from build123d import *
from build123d.topology import SkipClean

# Parameters (mm, degrees)
SKETCH1_R                                = 2.5
BOSS_EXTRUDE1_DEPTH                      = 2.5
SKETCH4_W                                = 130
SKETCH4_H                                = 30
BOSS_EXTRUDE2_DEPTH                      = 5
FILLET1_R                                = 10
FILLET2_R                                = 12.5
SKETCH5_R                                = 2.15
CUT_EXTRUDE1_DEPTH                       = 10
BOSS_EXTRUDE3_DEPTH                      = 2.5
LPATTERN1_COUNT                          = 2
LPATTERN1_PITCH                          = 23
MIRROR4_COPY_1_DEPTH                     = 2.5
MIRROR4_AT_THE_SECOND_PLANE_COPY_1_DEPTH = 2.5
MIRROR4_AT_THE_SECOND_PLANE_COPY_2_DEPTH = 2.5
MIRROR4_AT_THE_SECOND_PLANE_COPY_3_DEPTH = 2.5


with BuildPart() as part:
    # Sketch1 → Boss-Extrude1 (new, symmetric)
    with BuildSketch(Plane.XY):
        with BuildLine():
            ThreePointArc((-38.614160498, -3.933326056), (-23.874667518, 3.933250754), (-9.779272654, -5.036449778))
            ThreePointArc((-9.779272654, -5.036449778), (-5.727087063, -9.391510729), (0, -11))
            Line((0, -11), (0, -4))
            ThreePointArc((0, -4), (-4, 0), (0, 4))
            Line((0, 4), (0, 11))
            Line((0, 11), (-52.5, 11))
            Line((-52.5, 11), (-52.5, 0))
            ThreePointArc((-52.5, 0), (-47.044040574, -7.216086067), (-38.614160498, -3.933326056))
        make_face()
        with Locations((-45, 0)):
            Circle(SKETCH1_R, mode=Mode.SUBTRACT)
    boss_extrude1 = extrude(amount=BOSS_EXTRUDE1_DEPTH, both=True)

    # Mirror1: Boss-Extrude1 across plane
    with SkipClean():  # the faces are left unmerged after this step: merging them gives an invalid solid
        add(boss_extrude1.mirror(Plane(origin=(0, 0, -2.5), x_dir=(0, 0, 1), z_dir=(-1, 0, 0))))

    # Sketch4 → Boss-Extrude2 (add)
    with SkipClean():  # the faces are left unmerged after this step: merging them gives an invalid solid
        with BuildSketch(Plane(origin=(0, 11, 0), x_dir=(1, 0, 0), z_dir=(0, 1, 0))):
            Rectangle(SKETCH4_W, SKETCH4_H)
        extrude(amount=BOSS_EXTRUDE2_DEPTH)

    # Fillet1
    fillet1_edges = [part.edges().sort_by_distance(p)[0] for p in [
        (-65, 13.5, -15),
        (-65, 13.5, 15),
        (65, 13.5, 15),
        (65, 13.5, -15),
    ]]
    fillet(fillet1_edges, radius=FILLET1_R)

    # Fillet2
    # the kernel refuses this fillet: 12.5 mm, written as the material it adds along each edge
    with BuildSketch(Plane(origin=(-52.5, 11, -2.5), x_dir=(-1, 0, 0), z_dir=(0, 0, 1))) as fillet2_piece_1:
        with BuildLine():
            CenterArc((12.443670675, 12.5), FILLET2_R, 184.301222305, 85.698777695)
            Line((-0.021123497, 11.5625), (-1.267602914, 11.46875))
            ThreePointArc((-1.267602914, 11.46875), (-1.25, 11), (-1.25, 0))
            Line((-1.25, 0), (0, -1.25))
            Line((0, -1.25), (12.443670675, -1.25))
            Line((12.443670675, -1.25), (12.443670675, 0))
        make_face()
    extrude(amount=5)
    with BuildSketch(Plane(origin=(52.5, 11, -2.5), x_dir=(1, 0, 0), z_dir=(0, 0, 1))) as fillet2_piece_2:
        with BuildLine():
            CenterArc((12.443670675, -12.5), FILLET2_R, 90, 85.698777695)
            Line((-0.021123497, -11.5625), (-1.267602914, -11.46875))
            ThreePointArc((-1.267602914, -11.46875), (-1.25, -11), (-1.25, 0))
            Line((-1.25, 0), (0, 1.25))
            Line((0, 1.25), (12.443670675, 1.25))
            Line((12.443670675, 1.25), (12.443670675, 0))
        make_face()
    extrude(amount=5)

    # Sketch5 → Cut-Extrude1 (cut)
    with BuildSketch(Plane(origin=(0, 16, 0), x_dir=(1, 0, 0), z_dir=(0, 1, 0))):
        with Locations(Location((-57, -8, 0), (0, 0, 180))):
            Circle(SKETCH5_R)
        with Locations(Location((-57, 8, 0), (0, 0, 180))):
            Circle(SKETCH5_R)
        with Locations(Location((-23, -8, 0), (0, 0, 180))):
            Circle(SKETCH5_R)
        with Locations(Location((-23, 8, 0), (0, 0, 180))):
            Circle(SKETCH5_R)
    cut_extrude1 = extrude(amount=-CUT_EXTRUDE1_DEPTH, mode=Mode.SUBTRACT)

    # Mirror2: Cut-Extrude1 across plane
    add(cut_extrude1.mirror(Plane(origin=(0, 0, 0), x_dir=(0, 0, 1), z_dir=(1, 0, 0))), mode=Mode.SUBTRACT)

    # Sketch7 → Boss-Extrude3 (add, symmetric)
    with BuildSketch(Plane(origin=(36.5, 0, 0), x_dir=(0, 0, -1), z_dir=(1, 0, 0))):
        Polygon((5, 11), (2.5, 11), (2.5, 6), (7.5, 11), align=None)
    boss_extrude3 = extrude(amount=BOSS_EXTRUDE3_DEPTH, both=True)

    # LPattern1: Boss-Extrude3 ×2
    with Locations(*[(-i * LPATTERN1_PITCH, 0, 0) for i in range(1, LPATTERN1_COUNT)]):
        add(boss_extrude3)

    # Mirror4: Boss-Extrude3 across plane
    add(boss_extrude3.mirror(Plane.XY))

    # Mirror4 copy 1 sketch → Mirror4 copy 1 (add, symmetric)
    with BuildSketch(Plane(origin=(13.5, 0, 0), x_dir=(0, 0, 1), z_dir=(1, 0, 0))):
        Polygon((5, -11), (2.5, -11), (2.5, -6), (7.5, -11), align=None)
    extrude(amount=MIRROR4_COPY_1_DEPTH, both=True)

    # Mirror4 at the second plane: Boss-Extrude3 across plane
    add(boss_extrude3.mirror(Plane(origin=(0, 0, 0), x_dir=(0, 0, 1), z_dir=(1, 0, 0))))

    # Mirror4 at the second plane copy 1 sketc → Mirror4 at the second plane copy 1 (add, symmetric)
    with BuildSketch(Plane(origin=(-13.5, 0, 0), x_dir=(0, 0, -1), z_dir=(-1, 0, 0))):
        Polygon((5, -11), (2.5, -11), (2.5, -6), (7.5, -11), align=None)
    extrude(amount=MIRROR4_AT_THE_SECOND_PLANE_COPY_1_DEPTH, both=True)

    # Mirror4 at the second plane copy 2 sketc → Mirror4 at the second plane copy 2 (add, symmetric)
    with BuildSketch(Plane.ZY.offset(36.5)):
        Polygon((5, 11), (2.5, 11), (2.5, 6), (7.5, 11), align=None)
    extrude(amount=MIRROR4_AT_THE_SECOND_PLANE_COPY_2_DEPTH, both=True)

    # Mirror4 at the second plane copy 3 sketc → Mirror4 at the second plane copy 3 (add, symmetric)
    with BuildSketch(Plane.ZY.offset(13.5)):
        Polygon((5, 11), (2.5, 11), (2.5, 6), (7.5, 11), align=None)
    extrude(amount=MIRROR4_AT_THE_SECOND_PLANE_COPY_3_DEPTH, both=True)


solid = part.part
The listing builds one solid part. Answer for the finished solid, in the listing's coordinates (mm). A direction names the side the tool comes from. Coordinates: 2 decimals unless noted, no trailing zeros. Loops run counter-clockwise (first coordinate to the right, second up) from the corner with the lowest first, then second, coordinate; pieces in that order, holes last. Notation, with made-up numbers: (38, 73.25) -> (54, 73.25) arc R27 ccw to (54, 100.25) -> close; hole circle Ø3 at (-8, -28). An arc over 180 degrees is marked (long way). Answer in a Markdown table with one row per item. Add a question column.
1. The part is cut by section A-A, the plane x = 57. Write down the section's boundary in (y, z).
2. The part is cut by section C-C, the plane y = -9. Write down the section's boundary in (x, z), then the cut area to 3 significant figures.
3. Consider line 1 (Y direction, x = -29.5, z = -11); line 2 (Z direction, x = 10, y = 1.75); line 3 (Y direction, x = -42, z = -2). Determine where each line is inside the solid, lowest interval first. Write a range as [from, to].
4. Determine the mould class of faces 4 (the flat face through (1, 5, -2.5)), 5 (the flat face through (-16, 9, 4)), 6 (the cylindrical face through (54.85, 13.54, 8.09)) for opening direction Z: +Z half, -Z half, draft (parallel to the pull), parting line (faces both ways), or undercut.
5. The part is cut by section D-D, the plane z = 12.5. Write down the section's boundary in (x, y).
6. The part is cut by section B-B, the plane x = 22.5. Write down the section's boundary in (y, z).
7. Flat-ended cylindrical pins translate along their axes: P1, Ø6.5, axis at x = 13, y = 1.5, coming from the -Z side; P2, Ø1.5, axis at y = 8, z = -4, coming from the -X side; P3, Ø5.5, axis at x = 23, z = 8, coming from the -Y side. Find the tip coordinate at first contact, or state that the pin passes through.
8. For faces 1 (the flat face through (39, 9, -4)), 2 (the flat face through (34, 9, -4)), 3 (the cylindrical face through (-54.85, 13.54, -7.91)), determine the directions among +Z, -Z, +X, -X, +Y, -Y from which every point of the face is accessible in a straight line to the end or side of a thin tool.
Answer below:
| question | item | result |
|---|---|---|
| 1 | outline | (8.15, -2.5) -> (11, -2.5) -> (11, -5.85) -> (16, -5.85) -> (16, 5.85) -> (11, 5.85) -> (11, 2.5) -> (8.15, 2.5) -> close; (11, -14.8) -> (16, -14.8) -> (16, -10.15) -> (11, -10.15) -> close; (11, 10.15) -> (16, 10.15) -> (16, 14.8) -> (11, 14.8) -> close |
| 2 | outline | (-6.32, -2.5) -> (6.32, -2.5) -> (6.32, 2.5) -> (-6.32, 2.5) -> close |
| 2 | area | 63.2 mm2 |
| 3 | line 1 | [11, 16] |
| 3 | line 2 | [-2.5, 2.5] |
| 3 | line 3 | [-6.87, 16] |
| 4 | face 4 | -Z half |
| 4 | face 5 | draft |
| 4 | face 6 | undercut |
| 5 | outline | (-61.61, 11) -> (61.61, 11) -> (61.61, 16) -> (-61.61, 16) -> close |
| 6 | outline | (3.82, -2.5) -> (11, -2.5) -> (11, -5.91) -> (16, -5.91) -> (16, 5.91) -> (11, 5.91) -> (11, 2.5) -> (3.82, 2.5) -> close; (11, -15) -> (16, -15) -> (16, -10.09) -> (11, -10.09) -> close; (11, 10.09) -> (16, 10.09) -> (16, 15) -> (11, 15) -> close |
| 7 | P1 | z = -2.5 |
| 7 | P2 | x = -39 |
| 7 | P3 | y = 11 |
| 8 | face 1 | -Z, +X, -Y |
| 8 | face 2 | -Z, -Y |
| 8 | face 3 | +Y, -Y |
